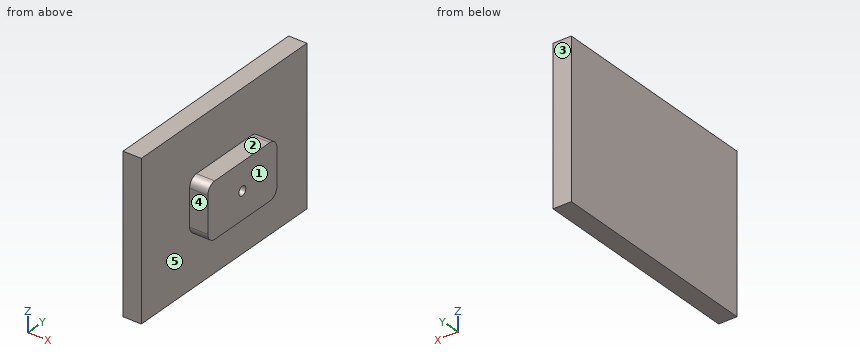
```python
from build123d import *

# Parameters (mm, degrees)
F0_W     = 120
F0_H     = 85
F0_W_2   = 50
F0_H_2   = 30
F1_DEPTH = 10
F2_DEPTH = 20
F3_R     = 2.5
F4_DEPTH = 10
F5_R     = 5


with BuildPart() as f1:
    # F0 (on Right) → F1 (new body)
    with BuildSketch(Plane.YZ):
        Rectangle(F0_W, F0_H)
        Rectangle(F0_W_2, F0_H_2, mode=Mode.SUBTRACT)
        Rectangle(F0_W_2, F0_H_2)
    extrude(amount=F1_DEPTH)

    # F0 (on Right) → F2 (join)
    with BuildSketch(Plane.YZ):
        Rectangle(F0_W_2, F0_H_2)
    extrude(amount=F2_DEPTH)

    # F3 (on face) → F4 (cut)
    with BuildSketch(Plane.YZ.offset(20)):
        Circle(F3_R)
    extrude(amount=-F4_DEPTH, mode=Mode.SUBTRACT)

    # F5
    f5_edges = [f1.edges().sort_by_distance(p)[0] for p in [
        (15, -25, 15),
        (15, 25, 15),
        (15, -25, -15),
        (15, 25, -15),
    ]]
    fillet(f5_edges, radius=F5_R)


solid = f1.part
```
The model under review builds one solid part; all positions refer to its coordinate system, in mm. Face numbers are marked on the shaded views. A direction names the side the tool comes from. Give positions to 0.01 mm unless a question says otherwise; leave off trailing zeros. Order: outer loops, then holes, each group sorted by start corner. A loop starts at its lowest first (then second) coordinate and runs counter-clockwise, first axis right, second up. Notation, with made-up numbers: (-25.75, -13) - (32.25, -13) arc R23 ccw to (32.25, 3) - close; hole circle Ø5 at (-2, 12.25). An arc over 180 degrees is marked (long way). Use CSV: the item, a comma, the result in double quotes. Start each with the question number.
Q1. Clearance check with flat-ended pins moving along their axes: pin 1 Ø3 at (x, z) = (15, -4) entering from +Y; pin 2 Ø10 at (y, z) = (-22.5, -30.5) entering from -X; pin 3 Ø1.5 at (y, z) = (-0.5, 0.5) entering from +X; pin 4 Ø8 at (x, z) = (16.5, 4) entering from -Y. State where each tip first meets the part, or that it passes through.
Q2. The part is to be moulded in two halves that separate along Y. For the marked faces 3, 4 and 5, say which applies: +Y half, -Y half, draft (parallel to the pull), parting line (faces both ways), or undercut.
Q3. Tool access review of the marked faces 1 and 2: name each direction out of +Z, -Z, +X, -X, +Y, -Y from which nothing blocks a thin tool from reaching the whole face with its end or side.
Q4. To check wall thickness, follow line 1 along Z through (x, y) = (16.75, 0); line 2 along X through (y, z) = (-16.5, 22); line 3 along Y through (x, z) = (17, -3). State the ranges of each line that lie inside material, in increasing order. Write a range as [from, to].
Q5. We need section C-C, the plane y = 0. Write out the cut boundary in (x, z), and give its area (3 significant figures).
Q6. We need section D-D, the plane z = -23. Write out the cut boundary in (x, y), and give its area (3 significant figures).
Q7. We need section B-B, the plane z = 0. Write out the cut boundary in (x, y), and give its area (3 significant figures).
Q8. We need section A-A, the plane x = 13.75. Write out the cut boundary in (y, z).
Outcome:
1,pin 1,"stops at y = 25"
1,pin 2,"stops at x = 0"
1,pin 3,"stops at x = 10"
1,pin 4,"stops at y = -25"
2,face 3,"+Y half"
2,face 4,"-Y half"
2,face 5,"draft"
3,face 1,"+Z, -Z, +X, +Y, -Y"
3,face 2,"+Z, +X, +Y, -Y"
4,line 1,"z = [-15, -2.5], [2.5, 15]"
4,line 2,"x = [0, 10]"
4,line 3,"y = [-25, 25]"
5,outline,"(0, -42.5) - (10, -42.5) - (10, -15) - (20, -15) - (20, -2.5) - (10, -2.5) - (10, 2.5) - (20, 2.5) - (20, 15) - (10, 15) - (10, 42.5) - (0, 42.5) - close"
5,area,"1,100 mm^2"
6,outline,"(0, -60) - (10, -60) - (10, 60) - (0, 60) - close"
6,area,"1,200 mm^2"
7,outline,"(0, -60) - (10, -60) - (10, -25) - (20, -25) - (20, -2.5) - (10, -2.5) - (10, 2.5) - (20, 2.5) - (20, 25) - (10, 25) - (10, 60) - (0, 60) - close"
7,area,"1,650 mm^2"
8,outline,"(-25, -10) arc R5 ccw to (-20, -15) - (20, -15) arc R5 ccw to (25, -10) - (25, 10) arc R5 ccw to (20, 15) - (-20, 15) arc R5 ccw to (-25, 10) - close; hole circle Ø5 at (0, 0)"
